```python
from build123d import *

# Parameters (mm, degrees)
F2_R     = 5
F3_DEPTH = 5


with BuildPart() as f1:
    # F0 (on Front) → F1 (revolve)
    with BuildSketch(Plane.XZ):
        Polygon((-25, 25), (-25, 0), (-22.5, 0), (-22.5, 7.5), (-20, 7.5), (-20, 12.5), (-22.5, 12.5), (-22.5, 20), (-20, 20), (-20, 25), align=None)
        Polygon((-22.5, 0), (-25, 0), (-25, -25), (-20, -25), (-20, -20), (-22.5, -20), (-22.5, -12.5), (-20, -12.5), (-20, -7.5), (-22.5, -7.5), align=None)
    revolve(axis=Axis((0, 0, 7.500000298), (0, 0, -1)))

    # F2 (on face) → F3 (join)
    with BuildSketch(Plane.XY.offset(25)):
        with BuildLine():
            ThreePointArc((-22.9128784748, -10), (-25, 0), (-22.9128784748, 10))
            Line((-22.9128784748, 10), (-47.5, 10))
            ThreePointArc((-47.5, 10), (-49.267766953, 9.267766953), (-50, 7.5))
            Line((-50, 7.5), (-50, 0))
            Line((-50, 0), (-50, -7.5))
            ThreePointArc((-50, -7.5), (-49.267766953, -9.267766953), (-47.5, -10))
            Line((-47.5, -10), (-22.9128784748, -10))
        make_face()
        with Locations((-40, 0)):
            Circle(F2_R, mode=Mode.SUBTRACT)
    extrude(amount=-F3_DEPTH)

    # F4: F1 across plane


with BuildPart() as f1_1:
    add(f1.part)
    add(f1.part.mirror(Plane.YZ))

    # F5: F1 across plane


with BuildPart() as f1_2:
    add(f1_1.part)
    add(f1_1.part.mirror(Plane.XY))


solid = f1_2.part
```
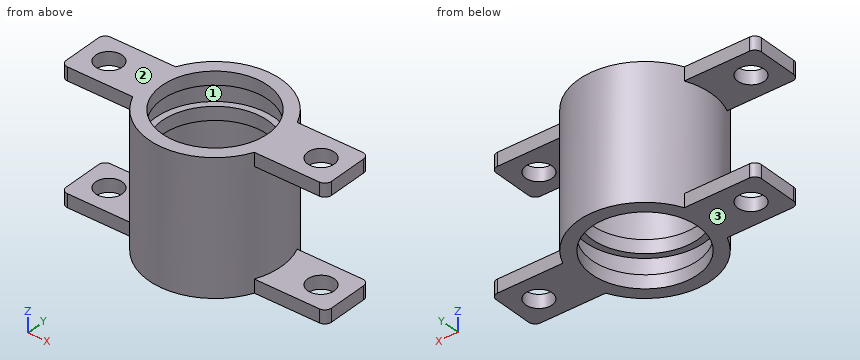
Work out the finished part from the listing and answer in its coordinate system (mm). Face numbers are marked on the shaded views. Give positions to 0.01 mm unless a question says otherwise; leave off trailing zeros. Order: outer loops, then holes, each group sorted by start corner. A loop starts at its lowest first (then second) coordinate and runs counter-clockwise, first axis right, second up. Notation, with made-up numbers: (-12, 74.5) -> (-6, 74.5) arc R29 cw to (-6, 109.5) -> close; hole circle Ø5 at (-23, -22). An arc over 180 degrees is marked (long way). Answer as CSV lines item,"result". Start each with the question number.
(1) Consider line 1 along Z through (x, y) = (-15.5, -15); line 2 along Y through (x, z) = (-40, -23.15); line 3 along Z through (x, y) = (-28, -5). Determine where each line is inside the solid, lowest interval first.
(2) For a pull along Z with two mould halves and no side action, classify the marked faces 1, 2 and 3 as released by +Z, released by -Z, zero draft, split by the parting line, or undercut.
(3) Section B-B, the plane x = -40 is taken. Write down the section's boundary in (y, z).
(4) Section D-D, the plane y = 0 is taken. Give the number of separate pieces and of enclosed holes in the cut face, plus the area to 3 significant figures.
(5) Each of these flat-tipped pins is pushed along its axis until it touches: pin 1 Ø9 at (x, y) = (40, 0) entering from -Z; pin 2 Ø2.5 at (x, z) = (-40, -22.5) entering from +Y; pin 3 Ø1.5 at (y, z) = (-16.5, 7) entering from -X; pin 4 Ø11.5 at (x, y) = (-40, 0) entering from -Z. Where does it stop, or does it pass through?
(6) Section A-A, the plane x = 29 is taken. Write down the section's boundary in (y, z).
(7) Section C-C, the plane z = -9 is taken. Write down the section's boundary in (x, y).
Entries:
1,line 1,"-25 to -20, -12.5 to -7.5, 7.5 to 12.5, 20 to 25"
1,line 2,"-10 to -5, 5 to 10"
1,line 3,"-25 to -20, 20 to 25"
2,face 1,"undercut"
2,face 2,"released by +Z"
2,face 3,"released by -Z"
3,outline,"(-10, -25) -> (-5, -25) -> (-5, -20) -> (-10, -20) -> close; (-10, 20) -> (-5, 20) -> (-5, 25) -> (-10, 25) -> close; (5, -25) -> (10, -25) -> (10, -20) -> (5, -20) -> close; (5, 20) -> (10, 20) -> (10, 25) -> (5, 25) -> close"
4,separate pieces,"6"
4,enclosed holes,"0"
4,area,"650 mm²"
5,pin 1,"through"
5,pin 2,"y = 10"
5,pin 3,"x = -19.41"
5,pin 4,"z = -25"
6,outline,"(-10, -25) -> (10, -25) -> (10, -20) -> (-10, -20) -> close; (-10, 20) -> (10, 20) -> (10, 25) -> (-10, 25) -> close"
7,outline,"circle Ø50 at (0, 0); hole circle Ø40 at (0, 0)"
